Autodesk Inventor part; units mm, degrees
ref_plane "YZ Plane" through (0, 0, 0) normal (1, 0, 0) x (0, 1, 0)
ref_plane "XZ Plane" through (0, 0, 0) normal (0, 1, 0) x (-1, 0, 0)
ref_plane "XY Plane" through (0, 0, 0) normal (0, 0, 1) x (1, 0, 0)
sketch "Skizze1" plane through (0, 0, 0) normal (0, 0, 1) x (1, 0, 0)
  circle A0 centre (0, 0) radius 1.65
  circle A1 centre (0, 0) radius 4.15 construction
  line L0 (0, 4.15) -> (3.9469, 1.2824)
  line L1 (3.9469, 1.2824) -> (2.4393, -3.3574)
  line L2 (2.4393, -3.3574) -> (-2.4393, -3.3574)
  line L3 (-2.4393, -3.3574) -> (-3.9469, 1.2824)
  line L4 (-3.9469, 1.2824) -> (0, 4.15)
  circle A2 centre (0, 0) radius 4.5
  dimension "d1" = 8.3
  dimension "d0" = 3.3
  dimension "d2" = 9
extrude "Extrusion1" add sketch "Skizze1" along normal blind 180 contours L0 L1 L2 L3 L4 | A2
extrude "Extrusion2" add sketch "Skizze1" against normal blind 9 contours L0 L1 L2 L3 L4
extrude "Extrusion3" add sketch "Skizze1" along normal blind 9 from surface at 180 contours L0 L1 L2 L3 L4
properties part number "Rod"
Geometry: final body of the model. Coordinates: model frame, mm. A direction names the side the tool comes from. Coordinates: 2 decimals unless noted, no trailing zeros. Order: outer loops, then holes, each group sorted by start corner. A loop starts at its lowest first (then second) coordinate and runs counter-clockwise, first axis right, second up. Notation, with made-up numbers: (60, 27.25) - (76, 27.25) arc R22 cw to (76, 59.25) - close; hole circle Ø4 at (33.5, 79.5). An arc over 180 degrees is marked (long way). Return JSON: item names as keys, results as strings. Group by question number.
1. Pull-direction query (Y, two-part tool) for faces 1 (the face through (-1.216, -1.115, 88.614)), 2 (the face through (2, 0, -9)), 3 (the face through (-2.001, 2.696, 184.437)); classes: pulls with the +Y half, pulls with the -Y half, needs draft (parallel to the pull), parting line crosses it, or undercut.
2. Cut plane A-A (z = 157). Output: boundary loops of the cut face in (x, y), plus the area to 3 significant figures.
3. Material intervals for line 1 along Y through (x, z) = (0, 107); line 2 along X through (y, z) = (0.25, 94); line 3 along Z through (x, y) = (-3.75, -2.25), sorted ascending. Write a range as [from, to].
4. Set-up query: faces 4 (the face through (3.2, -1.01, 184.44)), 5 (the face through (-3.183, -1.07, -4.437)), 6 (the face through (0, -3.357, 184)), 7 (the face through (-2.001, 2.696, -4.437)), 8 (the face through (3.2, -1.01, -4.44)). Return all of +Z, -Z, +X, -X, +Y, -Y with unobstructed straight access to the full face (end or side cutting, diameter ignored); none if empty.
5. Pin query (flat end, axial travel): pin 1 (1.5 mm diameter, centred on x = 1, z = -6.5, fed in from -Y); pin 2 (1 mm diameter, centred on y = 1, z = 32.5, fed in from +X); pin 3 (1 mm diameter, centred on x = -3.5, y = -2, fed in from +Z); pin 4 (2.5 mm diameter, centred on x = 0, y = 0, fed in from +Z). Return the tip coordinate at first contact, or that it passes through.
Resolved:
{
 "1": {"face 1": "undercut", "face 2": "needs draft", "face 3": "pulls with the +Y half"},
 "2": {"outline": "circle Ø9 at (0, 0); hole circle Ø3.3 at (0, 0)", "area": "55.1 mm²"},
 "3": {"line 1": "y = [-4.5, -1.65], [1.65, 4.5]", "line 2": "x = [-4.49, -1.63], [1.63, 4.49]", "line 3": "z = [0, 180]"},
 "4": {"face 4": "+Z, +X, -Y", "face 5": "-Z, -X, -Y", "face 6": "+Z, +X, -X, -Y", "face 7": "-Z, -X, +Y", "face 8": "-Z, +X, -Y"},
 "5": {"pin 1": "stops at y = -3.36", "pin 2": "stops at x = 4.47", "pin 3": "stops at z = 180", "pin 4": "passes through"}
}
